from build123d import *

# Parameters (mm, degrees)
F1_DEPTH = 15
F2_W     = 60
F2_H     = 30
F3_DEPTH = 10
F4_R     = 3.836856
F5_DEPTH = 25


with BuildPart() as f1:
    # F0 (on Top) → F1 (new body)
    with BuildSketch(Plane.XY):
        with BuildLine():
            Line((5.510565, 0), (0, 0))
            Line((0, 0), (0, -60))
            Line((0, -60), (5.815111, -60))
            ThreePointArc((5.815111, -60), (17.941032, -36.85211), (30.066952, -60))
            Line((30.066952, -60), (35, -60))
            Line((35, -60), (35, 0))
            Line((35, 0), (29.736414, 0))
            ThreePointArc((29.736414, 0), (17.62349, -23.166624), (5.510565, 0))
        make_face()
    extrude(amount=F1_DEPTH)

    # F2 (on face) → F3 (join)
    with BuildSketch(Plane.YZ.offset(35)):
        with Locations((-30, 15)):
            Rectangle(F2_W, F2_H)
    extrude(amount=F3_DEPTH)

    # F4 (on face) → F5 (cut)
    with BuildSketch(Plane(origin=(35, 0, 0), x_dir=(0, -1, 0), z_dir=(-1, 0, 0))):
        with Locations((10.00252, 22.384789)):
            Circle(F4_R)
        with Locations((30.00252, 22.384789)):
            Circle(F4_R)
        with Locations((50.00252, 22.384789)):
            Circle(F4_R)
    extrude(amount=-F5_DEPTH, mode=Mode.SUBTRACT)


solid = f1.part
Part model, mm, in its own coordinate system. A direction names the side the tool comes from. Round coordinates to 2 decimals unless told otherwise and drop trailing zeros. Loops run counter-clockwise (first coordinate to the right, second up) from the corner with the lowest first, then second, coordinate; pieces in that order, holes last. Notation, with made-up numbers: (54, -6) - (97, -6) arc R19 cw to (97, 10) - close; hole circle Ø6 at (-7.75, -18). An arc over 180 degrees is marked (long way). Answer as a JSON object with one key per item and string values.
Item 1: Band-saw the part on B-B on x = 36. List the corners of the cut face in (y, z), plus the area to 3 significant figures.
Output:
{"outline": "(-60, 0) - (0, 0) - (0, 30) - (-60, 30) - close; hole circle Ø7.67 at (-50, 22.38); hole circle Ø7.67 at (-30, 22.38); hole circle Ø7.67 at (-10, 22.38)", "area": "1,660 mm2"}
Item 2: Pin check, flat tips, straight feed: pin 1 (7 mm diameter, centred on y = -30, z = 22.38, fed in from +X); pin 2 (12.5 mm diameter, centred on y = -10, z = 22.38, fed in from -X); pin 3 (6 mm diameter, centred on x = 9, z = 6.5, fed in from -Y); pin 4 (3 mm diameter, centred on y = -17, z = 8, fed in from -X). Stop position of each tip, or through.
Output:
{"pin 1": "through", "pin 2": "x = 35", "pin 3": "y = -42.94", "pin 4": "x = 0"}
Item 3: Pull direction Z, two halves, no side cores. Call faces 1 (the face through (39.93, -6.96, 20.05)), 2 (the face through (39.93, -46.96, 20.05)), 3 (the face through (39, 0, 15)), 4 (the face through (17, -30, 15)): pulls with the +Z half, pulls with the -Z half, needs draft (parallel to the pull), parting line crosses it, or undercut.
Output:
{"face 1": "undercut", "face 2": "undercut", "face 3": "needs draft", "face 4": "pulls with the +Z half"}
Item 4: Band-saw the part on D-D on y = -8. List the corners of the cut face in (x, z), plus the area to 3 significant figures.
Output:
{"outline": "(0, 0) - (2.88, 0) - (2.88, 15) - (0, 15) - close; (32.37, 0) - (45, 0) - (45, 19.11) - (35, 19.11) - (35, 15) - (32.37, 15) - close; (35, 25.66) - (45, 25.66) - (45, 30) - (35, 30) - close", "area": "317 mm2"}
Item 5: Band-saw the part on A-A on y = -30.5. List the corners of the cut face in (x, z), plus the area to 3 significant figures.
Output:
{"outline": "(0, 0) - (45, 0) - (45, 18.58) - (35, 18.58) - (35, 15) - (0, 15) - close; (35, 26.19) - (45, 26.19) - (45, 30) - (35, 30) - close", "area": "749 mm2"}
Item 6: Band-saw the part on C-C on z = 9. List the corners of the cut face in (x, y), plus the area to 3 significant figures.
Output:
{"outline": "(0, -60) - (5.82, -60) arc R14.75 cw (long way) to (30.07, -60) - (45, -60) - (45, 0) - (29.74, 0) arc R14.75 cw (long way) to (5.51, 0) - (0, 0) - close", "area": "1,550 mm2"}
Item 7: Tool access for faces 5 (the face through (35, -30, 28)), 6 (the face through (3, -60, 7)): list every direction of +Z, -Z, +X, -X, +Y, -Y with a clear straight run to the whole face (end or side of a thin tool).
Output:
{"face 5": "+Z, -X, +Y, -Y", "face 6": "+Z, -Z, +X, -X, -Y"}
Item 8: Wall check: L1, parallel to Z at x = 13, y = -24; L2, parallel to X at y = -47, z = 3.5; L3, parallel to X at y = -13.5, z = 20. Give the ranges that are in metal, low to high.
Output:
{"L1": "0 to 15", "L2": "0 to 3.93, 31.95 to 45", "L3": "35 to 45"}
